```python
from build123d import *

# Parameters (mm, degrees)
F0_R     = 1.5
F1_DEPTH = 1.5
F2_R     = 5
F3_R     = 2


with BuildPart() as f1:
    # F0 (on Top) → F1 (new body)
    with BuildSketch(Plane.XY):
        with BuildLine():
            Line((34.3576592932, -18), (20.9590200014, -3.3779510381))
            ThreePointArc((20.9590200014, -3.3779510381), (19.6454066855, 0), (20.9590200014, 3.3779510381))
            Line((20.9590200014, 3.3779510381), (34.3576592932, 18))
            Line((34.3576592932, 18), (18, 34.3576592932))
            Line((18, 34.3576592932), (18, 62))
            Line((18, 62), (10.9087121146, 62))
            ThreePointArc((10.9087121146, 62), (8.2084034903, 62.7918729423), (6.3634154002, 64.9166666667))
            ThreePointArc((6.3634154002, 64.9166666667), (0, 69), (-6.3634154002, 64.9166666667))
            ThreePointArc((-6.3634154002, 64.9166666667), (-8.2084034903, 62.7918729423), (-10.9087121146, 62))
            Line((-10.9087121146, 62), (-18, 62))
            Line((-18, 62), (-18, 34.3576592932))
            Line((-18, 34.3576592932), (-34.3576592932, 18))
            Line((-34.3576592932, 18), (-20.9590200014, 3.3779510381))
            ThreePointArc((-20.9590200014, 3.3779510381), (-19.6454066855, 0), (-20.9590200014, -3.3779510381))
            Line((-20.9590200014, -3.3779510381), (-34.3576592932, -18))
            Line((-34.3576592932, -18), (-18, -34.3576592932))
            Line((-18, -34.3576592932), (-18, -54))
            Line((-18, -54), (0, -60))
            Line((0, -60), (18, -54))
            Line((18, -54), (18, -34.3576592932))
            Line((18, -34.3576592932), (34.3576592932, -18))
        make_face()
        with Locations((-13, -44.75)):
            Circle(F0_R, mode=Mode.SUBTRACT)
        with Locations((-27.2708152802, -18.7855339059)):
            Circle(F0_R, mode=Mode.SUBTRACT)
        with Locations((-18.7855339059, -27.2708152802)):
            Circle(F0_R, mode=Mode.SUBTRACT)
        with Locations((-15.25, -15.25)):
            Circle(F0_R, mode=Mode.SUBTRACT)
        with Locations((13, -44.75)):
            Circle(F0_R, mode=Mode.SUBTRACT)
        with Locations((15.25, -15.25)):
            Circle(F0_R, mode=Mode.SUBTRACT)
        with Locations((18.7855339059, -27.2708152802)):
            Circle(F0_R, mode=Mode.SUBTRACT)
        with Locations((27.2708152802, -18.7855339059)):
            Circle(F0_R, mode=Mode.SUBTRACT)
        with Locations((-27.2708152802, 18.7855339059)):
            Circle(F0_R, mode=Mode.SUBTRACT)
        with Locations((-18.7855339059, 27.2708152802)):
            Circle(F0_R, mode=Mode.SUBTRACT)
        with Locations((-15.25, 15.25)):
            Circle(F0_R, mode=Mode.SUBTRACT)
        with Locations((-13, 57)):
            Circle(F0_R, mode=Mode.SUBTRACT)
        with Locations((15.25, 15.25)):
            Circle(F0_R, mode=Mode.SUBTRACT)
        with Locations((27.2708152802, 18.7855339059)):
            Circle(F0_R, mode=Mode.SUBTRACT)
        with Locations((18.7855339059, 27.2708152802)):
            Circle(F0_R, mode=Mode.SUBTRACT)
        with Locations((13, 57)):
            Circle(F0_R, mode=Mode.SUBTRACT)
    extrude(amount=F1_DEPTH)

    # F2
    f2_edges = [f1.edges().sort_by_distance(p)[0] for p in [
        (-18, -54, 0.75),
        (0, -60, 0.75),
        (18, -54, 0.75),
        (-18, 62, 0.75),
        (-18, 34.357659, 0.75),
        (-18, -34.357659, 0.75),
        (18, -34.357659, 0.75),
        (18, 34.357659, 0.75),
        (18, 62, 0.75),
    ]]
    fillet(f2_edges, radius=F2_R)

    # F3
    f3_edges = [f1.edges().sort_by_distance(p)[0] for p in [
        (-34.357659, -18, 0.75),
        (-34.357659, 18, 0.75),
        (34.357659, 18, 0.75),
        (34.357659, -18, 0.75),
    ]]
    fillet(f3_edges, radius=F3_R)


solid = f1.part
```
Geometry check sheet. Reference: the model listing, model coordinates, mm. A direction names the side the tool comes from. Round coordinates to 2 decimals unless told otherwise and drop trailing zeros. Loops run counter-clockwise (first coordinate to the right, second up) from the corner with the lowest first, then second, coordinate; pieces in that order, holes last. Notation, with made-up numbers: M 66,23 L 101,23 A11 ccw 101,27 Z; hole C 7,76 d6. An arc over 180 degrees is marked long. Return JSON: item names as keys, results as strings. Group by question number.
(1) Go/stop test with a flat-tipped pin: pin 1 (2.5 mm diameter, centred on x = 18.79, y = 27.27, fed in from -Z). Record where the tip stops, or that it passes through.
(2) Section check B-B, the plane x = 23.5. Enter the section's corners in (y, z), and give its area (3 significant figures).
(3) Section check D-D, the plane x = -4. Enter the section's corners in (y, z), and give its area (3 significant figures).
(4) Mould release check, pull along Y, two halves, no side actions. Record for faces 3 (the face through (-16, 61, 1)), 4 (the face through (-25.84, -18.33, 0.74)), 5 (the face through (-26.33, -26.03, 0.74)), 6 (the face through (27.1, -10.08, 0.74)): pulls with the +Y half, pulls with the -Y half, needs draft (parallel to the pull), parting line crosses it, or undercut.
(5) Scan lines: line 1 along Y through (x, z) = (26, 0.3); line 2 along X through (y, z) = (-45, 0.9); line 3 along X through (y, z) = (18, 1.25). Record each from-to range of solid material in increasing order. Write a range as [from, to].
(6) Section check A-A, the plane y = -15.25. Enter the section's corners in (x, z), and give its area (3 significant figures).
(7) Section check C-C, the plane y = 53. Enter the section's corners in (x, z).
(8) Set-up check for faces 1 (the face through (-13.325, -46.214, 0.74)), 2 (the face through (26.927, 9.891, 0.74)): record each of +Z, -Z, +X, -X, +Y, -Y from which the full face is reachable in a straight line by a thin tool's end or side.
Data:
{
 "1": {"pin 1": "through"},
 "2": {"outline": "M -28.86,0 L -6.15,0 L -6.15,1.5 L -28.86,1.5 Z; M 6.15,0 L 28.86,0 L 28.86,1.5 L 6.15,1.5 Z", "area": "68.1 mm²"},
 "3": {"outline": "M -58.67,0 L 67.74,0 L 67.74,1.5 L -58.67,1.5 Z", "area": "190 mm²"},
 "4": {"face 3": "pulls with the +Y half", "face 4": "undercut", "face 5": "pulls with the -Y half", "face 6": "undercut"},
 "5": {"line 1": "[-26.36, -19.58], [-17.99, -8.88], [8.88, 17.99], [19.58, 26.36]", "line 2": "[-18, -14.48], [-11.52, 11.52], [14.48, 18]", "line 3": "[-33.59, -28.55], [-25.99, 25.99], [28.55, 33.59]"},
 "6": {"outline": "M -31.84,0 L -16.75,0 L -16.75,1.5 L -31.84,1.5 Z; M -13.75,0 L 13.75,0 L 13.75,1.5 L -13.75,1.5 Z; M 16.75,0 L 31.84,0 L 31.84,1.5 L 16.75,1.5 Z", "area": "86.5 mm²"},
 "7": {"outline": "M -18,0 L 18,0 L 18,1.5 L -18,1.5 Z"},
 "8": {"face 1": "+Z, -Z", "face 2": "+Z, -Z, +X"}
}
